```python
from build123d import *

# Parameters (mm, degrees)
SKETCH1_R           = 12
SKETCH1_R_2         = 7
SKETCH1_R_3         = 5.5
BOSS_EXTRUDE1_DEPTH = 2.9
SKETCH1_3_R         = 7
SKETCH1_3_R_2       = 5.5
BOSS_EXTRUDE2_DEPTH = 10
SKETCH7_R           = 5.5
CUT_EXTRUDE10_DEPTH = 8
SKETCH8_R           = 6
SKETCH8_R_2         = 5.5
CUT_EXTRUDE11_DEPTH = 1.8


with BuildPart() as part:
    # Sketch1 → Boss-Extrude1 (new body)
    # profile 1 of 4: a face of its own
    with BuildSketch(Plane(origin=(0, 0, 0), x_dir=(1, 0, 0), z_dir=(0, 1, 0))):
        Circle(SKETCH1_R)
        Circle(SKETCH1_R_2, mode=Mode.SUBTRACT)
    # profile 2 of 4: a face of its own
    with BuildSketch(Plane(origin=(0, 0, 0), x_dir=(1, 0, 0), z_dir=(0, 1, 0))):
        with BuildLine():
            ThreePointArc((12, 0), (11.769423369, -2.341083842), (11.086554407, -4.592201147))
            Line((11.086554407, -4.592201147), (17.959269152, 12))
            Line((17.959269152, 12), (17.959269152, 12.01))
            ThreePointArc((17.959269152, 12.01), (15.033265896, 19.073996744), (7.969269152, 22))
            Line((7.969269152, 22), (-7.969269152, 22))
            ThreePointArc((-7.969269152, 22), (-15.033265896, 19.073996744), (-17.959269152, 12.01))
            Line((-17.959269152, 12.01), (-17.959269152, 12))
            Line((-17.959269152, 12), (-11.086554257, -4.59220151))
            ThreePointArc((-11.086554257, -4.59220151), (-2.341084035, 11.769423331), (12, 0))
        make_face()
    # profile 3 of 4: a face of its own
    with BuildSketch(Plane(origin=(0, 0, 0), x_dir=(1, 0, 0), z_dir=(0, 1, 0))):
        Circle(SKETCH1_R_2)
    # profile 4 of 4: a face of its own
    with BuildSketch(Plane(origin=(0, 0, 0), x_dir=(1, 0, 0), z_dir=(0, 1, 0))):
        Circle(SKETCH1_R_3)
    extrude(amount=BOSS_EXTRUDE1_DEPTH)

    # Sketch1_3 → Boss-Extrude2 (add)
    with BuildSketch(Plane(origin=(0, 0, 0), x_dir=(1, 0, 0), z_dir=(0, 1, 0))):
        with Locations(Location((0, 0, 0), (0, 0, 270))):
            Circle(SKETCH1_3_R)
        Circle(SKETCH1_3_R_2)
    extrude(amount=BOSS_EXTRUDE2_DEPTH)

    # Sketch7 → Cut-Extrude10 (cut)
    with BuildSketch(Plane(origin=(0, 10, 0), x_dir=(1, 0, 0), z_dir=(0, 1, 0))):
        with Locations(Location((0, 0, 0), (0, 0, 270))):
            Circle(SKETCH7_R)
    extrude(amount=-CUT_EXTRUDE10_DEPTH, mode=Mode.SUBTRACT)

    # Sketch8 → Cut-Extrude11 (cut)
    with BuildSketch(Plane(origin=(0, 9.8, 0), x_dir=(1, 0, 0), z_dir=(0, 1, 0))):
        with Locations(Location((0, 0, 0), (0, 0, 270))):
            Circle(SKETCH8_R)
        with Locations(Location((0, 0, 0), (0, 0, 270))):
            Circle(SKETCH8_R_2, mode=Mode.SUBTRACT)
    extrude(amount=-CUT_EXTRUDE11_DEPTH, mode=Mode.SUBTRACT)


solid = part.part
```
Work out the finished part from the listing and answer in its coordinate system (mm). A direction names the side the tool comes from. Give positions to 0.01 mm unless a question says otherwise; leave off trailing zeros. Loops run counter-clockwise (first coordinate to the right, second up) from the corner with the lowest first, then second, coordinate; pieces in that order, holes last. Notation, with made-up numbers: M 87,40 L 118,40 A32 cw 118,72 Z; hole C 58,25 d11. An arc over 180 degrees is marked long. One line per item, written item: value. Start each with the question number.
1. Find section C-C (z = -1.5). Give the vertices of the cut face in (x, y).
2. Find section B-B (y = 5). Give the vertices of the cut face in (x, z), and give its area (3 significant figures).
3. Determine the mould class of faces 4 (the face through (1.802, 8.913, 5.723)), 5 (the face through (-14.955, 1.43, -19.151)), 6 (the face through (0, 0, -9)), 7 (the face through (0, 2, 0)) for opening direction Z: released by +Z, released by -Z, zero draft, split by the parting line, or undercut.
4. Find section D-D (y = 9). Give the vertices of the cut face in (x, z).
5. Find the intervals of material crossed by probe 1 along X at (y, z) = (4.1, 0); probe 2 along X at (y, z) = (9, 0); probe 3 along Y at (x, z) = (1.5, -5.5), in increasing order.
6. Each of these flat-tipped pins is pushed along its axis until it touches: P1, Ø9.5, axis at x = 2, z = -1, coming from the +Y side; P2, Ø5, axis at x = 3, y = 5, coming from the +Z side; P3, Ø1, axis at y = 3, z = -5, coming from the -X side; P4, Ø4, axis at y = 3, z = 6.5, coming from the +X side. Where does it stop, or does it pass through?
7. Which of the six approach directions +Z, -Z, +X, -X, +Y, -Y give full straight-line access (tool end or side, diameter ignored) to faces 1 (the face through (-6.834, 6.4, -1.517)), 2 (the face through (0, 1, -22)), 3 (the face through (-5, 8, 3))?
8. Find section A-A (x = 0). Give the vertices of the cut face in (y, z).
Reported:
1. outline: M -13.61,0 L 13.61,0 L 13.61,2.9 L 6.84,2.9 L 6.84,10 L 5.29,10 L 5.29,9.8 L 5.81,9.8 L 5.81,8 L 5.29,8 L 5.29,2 L -5.29,2 L -5.29,8 L -5.81,8 L -5.81,9.8 L -5.29,9.8 L -5.29,10 L -6.84,10 L -6.84,2.9 L -13.61,2.9 Z
2. outline: C 0,0 d14; hole C 0,0 d11
2. area: 58.9 mm²
3. face 4: undercut
3. face 5: released by -Z
3. face 6: zero draft
3. face 7: undercut
4. outline: C 0,0 d14; hole C 0,0 d12
5. probe 1: x = -7 to -5.5, 5.5 to 7
5. probe 2: x = -7 to -6, 6 to 7
5. probe 3: y = 0 to 8, 9.8 to 10
6. P1: stops at y = 10
6. P2: stops at z = 11.89
6. P3: stops at x = -15.26
6. P4: stops at x = 11.12
7. face 1: +Y
7. face 2: -Z, +X, -X, +Y, -Y
7. face 3: none
8. outline: M 0,-22 L 2.9,-22 L 2.9,-7 L 10,-7 L 10,-5.5 L 9.8,-5.5 L 9.8,-6 L 8,-6 L 8,-5.5 L 2,-5.5 L 2,5.5 L 8,5.5 L 8,6 L 9.8,6 L 9.8,5.5 L 10,5.5 L 10,7 L 2.9,7 L 2.9,12 L 0,12 Z
